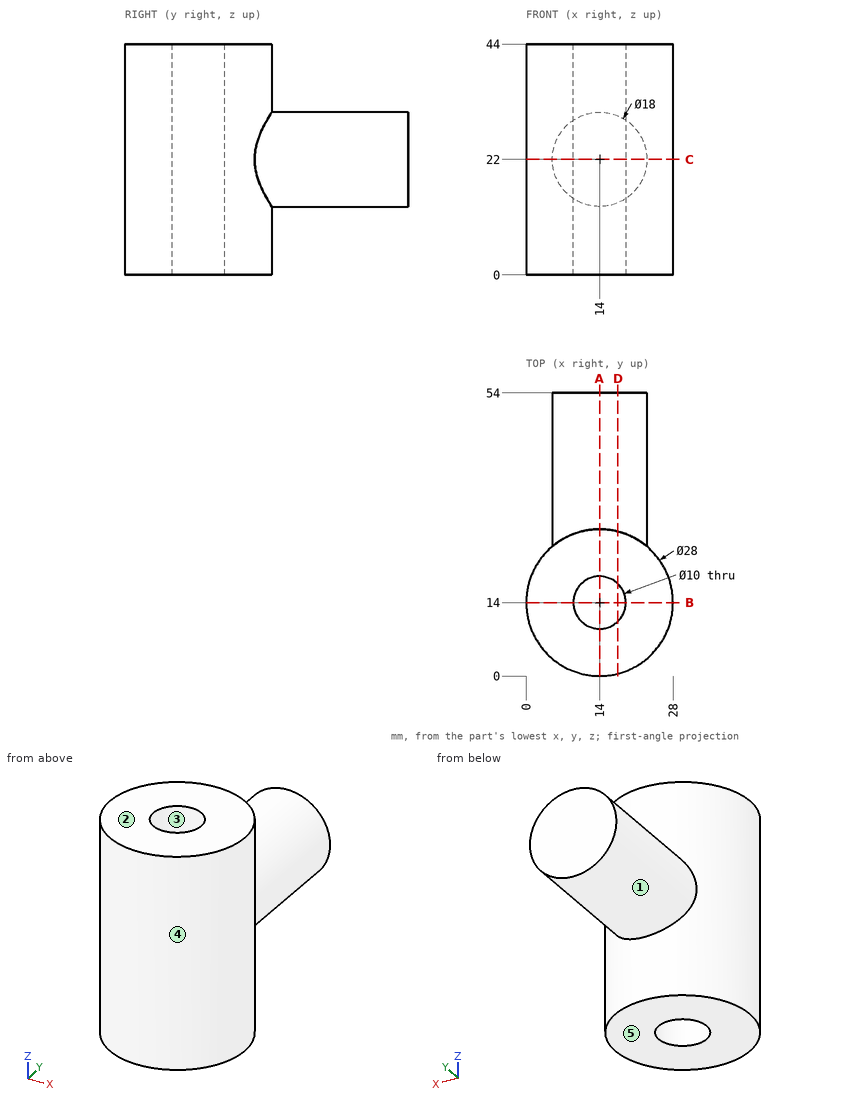
Geometry: see drawing. Coordinates: mm, zero at the bounding-box minimum. A direction names the side the tool comes from. Round coordinates to 2 decimals unless told otherwise and drop trailing zeros. Order: outer loops, then holes, each group sorted by start corner. A loop starts at its lowest first (then second) coordinate and runs counter-clockwise, first axis right, second up. Notation, with made-up numbers: (76.5, 61.5) - (118.5, 61.5) arc R18 ccw to (118.5, 72.5) - close; hole circle Ø1 at (64.25, -3). An arc over 180 degrees is marked (long way). One line per question, with ' | ' between items. Start each with the question number.
1) Cut plane A-A, the plane x = 14. Return the cut outline in (y, z), then the cut area to 3 significant figures.
2) Pull-direction query (Y, two-part tool) for the marked faces 3, 4 and 5; classes: +Y half, -Y half, draft (parallel to the pull), parting line (faces both ways), or undercut.
3) Ray query, probe 1 along Y at (x, z) = (14, 22.5); probe 2 along Y at (x, z) = (14, 32); probe 3 along X at (y, z) = (16, 13). Return the intervals inside material, ascending.
4) Contact query for flat-ended pins moving along their axis: P1, Ø1, axis at x = 14, y = 17, coming from the +Z side; P2, Ø3, axis at x = 7.5, y = 35, coming from the +Z side; P3, Ø1.5, axis at x = 18.5, z = 32, coming from the -Y side; P4, Ø1.5, axis at x = 21.5, z = 19, coming from the -Y side. Output: stop coordinate, or through.
5) Cut plane D-D, the plane x = 17.5. Return the cut outline in (y, z), then the cut area to 3 significant figures.
6) Set-up query: the marked faces 1 and 2. Return all of +Z, -Z, +X, -X, +Y, -Y with unobstructed straight access to the full face (end or side cutting, diameter ignored); none if empty.
7) Cut plane B-B, the plane y = 14. Return the cut outline in (x, z), then the cut area to 3 significant figures.
8) Cut plane C-C, the plane z = 22. Return the cut outline in (x, y).
Worked out:
1) outline: (0, 0) - (9, 0) - (9, 44) - (0, 44) - close; (19, 0) - (28, 0) - (28, 13) - (54, 13) - (54, 31) - (28, 31) - (28, 44) - (19, 44) - close | area: 1,260 mm^2
2) face 3: undercut | face 4: parting line | face 5: draft
3) probe 1: y = 0 to 9, 19 to 54 | probe 2: y = 0 to 9, 19 to 28 | probe 3: x = 0.14 to 9.42, 18.58 to 27.86
4) P1: passes through | P2: stops at z = 29.48 | P3: stops at y = 0.51 | P4: stops at y = 1.73
5) outline: (0.44, 0) - (10.43, 0) - (10.43, 44) - (0.44, 44) - close; (17.57, 0) - (27.56, 0) - (27.56, 13.71) - (54, 13.71) - (54, 30.29) - (27.56, 30.29) - (27.56, 44) - (17.57, 44) - close | area: 1,320 mm^2
6) face 1: +Y | face 2: +Z, +X, -X, +Y, -Y
7) outline: (0, 0) - (9, 0) - (9, 44) - (0, 44) - close; (19, 0) - (28, 0) - (28, 44) - (19, 44) - close | area: 792 mm^2
8) outline: (5, 24.72) arc R14 ccw (long way) to (23, 24.72) - (23, 54) - (5, 54) - close; hole circle Ø10 at (14, 14)
